Geometry: final body of the model. Coordinates: model frame, mm. A direction names the side the tool comes from. Coordinates: 2 decimals unless noted, no trailing zeros. Write item = value, one per line. Start each with the question number.
```python
from build123d import *

# Parameters (mm, degrees)
BASPROSKE_W             = 3
BASPROSKE_H             = 15.5
TOOTHCUT_DEPTH          = 23.12464689
TEETHCUTS_COUNT         = 60
TEETHCUTS_ANGLE         = 354
BORSKE_R                = 13
BORE_DEPTH              = 50.0000508
CROQUIS1_W              = 35.088386171
CROQUIS1_H              = 16.253421715
CORTAR_EXTRUIR1_DEPTH   = 23.10554405
SALIENTE_EXTRUIR1_DEPTH = 3


with BuildPart() as part:
    # BasProSke → Base-Revolve (revolve)
    with BuildSketch(Plane(origin=(0, 0, 0), x_dir=(1, 0, 0), z_dir=(0, 1, 0)), mode=Mode.PRIVATE) as base_revolve_sk:
        with Locations((1.5, 7.75)):
            Rectangle(BASPROSKE_W, BASPROSKE_H)
    revolve(base_revolve_sk.sketch.rotate(Axis((-10, 0, 0), (1, 0, 0)), 180), axis=Axis((-10, 0, 0), (1, 0, 0)))

    # TooCutSke → ToothCut (cut, through all)
    with BuildSketch(Plane(origin=(0, 0, 0), x_dir=(0, 0, -1), z_dir=(1, 0, 0))):
        with BuildLine():
            ThreePointArc((0.21493681, 14.372392917), (0, 14.374), (-0.21493681, 14.372392917))
            ThreePointArc((-0.21493681, 14.372392917), (-0.409732631, 14.953266942), (-0.662749221, 15.51124781))
            ThreePointArc((-0.662749221, 15.51124781), (0, 15.5254), (0.662749221, 15.51124781))
            ThreePointArc((0.662749221, 15.51124781), (0.409732631, 14.953266942), (0.21493681, 14.372392917))
        make_face()
    toothcut = extrude(amount=TOOTHCUT_DEPTH, mode=Mode.SUBTRACT)

    # TeethCuts: ToothCut ×60 about axis
    teethcuts_axis = Axis((-10, 0, 0), (1, 0, 0))
    for i in range(1, TEETHCUTS_COUNT):
        add(toothcut.rotate(teethcuts_axis, i * TEETHCUTS_ANGLE / (TEETHCUTS_COUNT - 1)), mode=Mode.SUBTRACT)

    # BorSke → Bore (cut, symmetric)
    with BuildSketch(Plane(origin=(0, 0, 0), x_dir=(0, 0, -1), z_dir=(1, 0, 0))):
        with Locations(Location((0, 0, 0), (0, 0, 180))):
            Circle(BORSKE_R)
    extrude(amount=BORE_DEPTH, both=True, mode=Mode.SUBTRACT)

    # Croquis1 → Cortar-Extruir1 (cut, through all)
    with BuildSketch(Plane(origin=(3, 0, 0), x_dir=(0, 0, -1), z_dir=(1, 0, 0))):
        with Locations((0.283547397, 8.126710858)):
            Rectangle(CROQUIS1_W, CROQUIS1_H)
    extrude(amount=-CORTAR_EXTRUIR1_DEPTH, mode=Mode.SUBTRACT)

    # Croquis2 → Saliente-Extruir1 (add, through all)
    with BuildSketch(Plane(origin=(3, 0, 0), x_dir=(0, 0, -1), z_dir=(1, 0, 0))):
        with BuildLine():
            Line((-13, 0), (-11.374, 0))
            ThreePointArc((-11.374, 0), (0, -11.374), (11.374, 0))
            Line((11.374, 0), (13, 0))
            ThreePointArc((13, 0), (0, -13), (-13, 0))
        make_face()
    extrude(amount=-SALIENTE_EXTRUIR1_DEPTH)


solid = part.part
```
Item 1: Draft query along Z for faces 5 (the flat face through (0, -12, 0)), 6 (the cylindrical face through (1.479, -11.854, 9.116)), 7 (the cylindrical face through (1.479, -1.157, 14.909)). Return one class per face: pulls with the +Z half, pulls with the -Z half, needs draft (parallel to the pull), parting line crosses it, or undercut.
Item 2: First-contact query: pin 1 (1 mm diameter, centred on x = 1.5, y = -11.5, fed in from +Z); pin 2 (1 mm diameter, centred on x = 2, y = -13, fed in from -Z). Flat tips, straight axial feed; report the tip coordinate or a pass-through.
Item 3: Material intervals for probe 1 along Z at (x, y) = (1.25, -5); probe 2 along Z at (x, y) = (1.05, -10.25); probe 3 along Y at (x, z) = (1.35, -12), sorted ascending. Write a range as [from, to].
Item 4: Reachability of faces 1 (the cylindrical face through (1.479, -7.827, -12.742)), 2 (the cylindrical face through (1.48, -14.08, -5)), 3 (the cylindrical face through (1.48, -11.38, -9.7)), 4 (the cylindrical face through (1.48, -7.81, 12.73)) from +Z, -Z, +X, -X, +Y, -Y: full face, straight path, thin tool, end or side. Return the list, or none.
Ans:
q1.face_5 = needs draft
q1.face_6 = undercut
q1.face_7 = pulls with the +Z half
q2.pin_1 = 10.92
q2.pin_2 = -8.58
q3.probe_1 = [-14.08, -10.22], [10.22, 14.08]
q3.probe_2 = [-10.81, -4.93], [4.93, 10.81]
q3.probe_3 = [-9.81, -9.36], [-8.36, 0]
q4.face_1 = -Z, +X, -X
q4.face_2 = +X, -X, -Y
q4.face_3 = +X, -X
q4.face_4 = +Z, +X, -X
